Build history of the part. All positions in model axes, mm. Coordinates: 2 decimals unless noted, no trailing zeros. Order: outer loops, then holes, each group sorted by start corner. A loop starts at its lowest first (then second) coordinate and runs counter-clockwise, first axis right, second up. Notation, with made-up numbers: (-3.5, 11) - (40.5, 11) arc R21 cw to (40.5, 49) - close; hole circle Ø1 at (46, 46). An arc over 180 degrees is marked (long way). One line per item, written item: value.
Autodesk Inventor part; units mm, degrees
ref_plane "YZ Plane" through (0, 0, 0) normal (1, 0, 0) x (0, 1, 0)
ref_plane "XZ Plane" through (0, 0, 0) normal (0, 1, 0) x (-1, 0, 0)
ref_plane "XY Plane" through (0, 0, 0) normal (0, 0, 1) x (1, 0, 0)
sketch "Эскиз1" plane through (0, 0, 0) normal (1, 0, 0) x (0, 1, 0)
  circle A0 centre (0, 0) radius 14
  dimension "d0" = 28
extrude "Выдавливание1" add sketch "Эскиз1" along normal mid plane 45
sketch "Эскиз2" plane through (22.5, 0, 0) normal (1, 0, 0) x (0, 0, -1)
  point P0 (0, 0)
  point P1 (0, 0)
hole "Отверстие1" at (22.5, 0, 0) direction (-1, 0, 0) diameter 6 depth 60
fillet "Сопряжение1" radius 0.1 2 edges at (-22.5, 0, 3) (22.5, 0, 3)
properties part number "Вал конвейера 2"
1. Band-saw the part on A-A, the plane z = 0. Give the cut face in (x, y).
Values found:
outline: (-22.5, -14) - (22.5, -14) - (22.5, -3.1) arc R0.1 ccw to (22.4, -3) - (-22.4, -3) arc R0.1 ccw to (-22.5, -3.1) - close; (-22.5, 3.1) arc R0.1 ccw to (-22.4, 3) - (22.4, 3) arc R0.1 ccw to (22.5, 3.1) - (22.5, 14) - (-22.5, 14) - close
2. Two-plate mould, pull along Y, no slides. Class faces 1 (the face through (-22.5, -0.2, 3.3)), 2 (the face through (0.315, 12.932, -5.362)), 3 (the face through (0, 0, 3)): pulls with the +Y half, pulls with the -Y half, needs draft (parallel to the pull), parting line crosses it, or undercut.
Values found:
face 1: needs draft
face 2: parting line crosses it
face 3: undercut
3. Probe line 1 along Y through (x, z) = (14, -0.25); line 2 along Z through (x, y) = (-1, 0); line 3 along Y through (x, z) = (5.5, 2.5). List the from-to ranges inside material, lowest first.
Values found:
line 1: y = -14 to -2.99, 2.99 to 14
line 2: z = -14 to -3, 3 to 14
line 3: y = -13.77 to -1.66, 1.66 to 13.77
4. Flat gauge pins, fed straight in: P1, Ø1.5, axis at x = 7.5, z = 3, coming from the +Y side; P2, Ø4, axis at x = 3, z = -7, coming from the +Y side; P3, Ø1.5, axis at x = -1, y = 10, coming from the -Z side. Where does each tip first touch, or does it go through?
Values found:
P1: stops at y = 13.82
P2: stops at y = 13.08
P3: stops at z = -10.51
5. Band-saw the part on C-C, the plane x = -5.5. Give the cut face in (y, z).
Values found:
outline: circle Ø28 at (0, 0); hole circle Ø6 at (0, 0)
6. Band-saw the part on D-D, the plane y = -11.5. Give the cut face in (x, z).
Values found:
outline: (-22.5, -7.98) - (22.5, -7.98) - (22.5, 7.98) - (-22.5, 7.98) - close
